from build123d import *

# Parameters (mm, degrees)
F0_W      = 16
F0_H      = 16
F1_DEPTH  = 16
F2_R      = 1
F4_R      = 1.5
F5_DEPTH  = 1
F3_R      = 1.5
F6_DEPTH  = 1
F7_R      = 1.5
F8_DEPTH  = 1
F9_R      = 1.5
F10_DEPTH = 1
F12_R     = 1.5
F13_DEPTH = 1
F11_R     = 1.5
F14_DEPTH = 1


with BuildPart() as f1:
    # F0 (on Top) → F1 (new body)
    with BuildSketch(Plane.XY):
        Rectangle(F0_W, F0_H)
    extrude(amount=F1_DEPTH)

    # F2
    f2_edges = [f1.edges().sort_by_distance(p)[0] for p in [
        (8, 0, 0),
        (8, 8, 8),
        (8, -8, 8),
        (8, 0, 16),
        (-8, 0, 16),
        (-8, 0, 0),
        (-8, -8, 8),
        (-8, 8, 8),
        (0, -8, 16),
        (0, -8, 0),
        (0, 8, 0),
        (0, 8, 16),
    ]]
    fillet(f2_edges, radius=F2_R)

    # F4 (on face) → F5 (cut)
    with BuildSketch(Plane.XY.offset(16)):
        with Locations((3.670213, -3.041311)):
            Circle(F4_R)
        with Locations((3.670213, 2.806282)):
            Circle(F4_R)
        with Locations((0, 2.806282)):
            Circle(F4_R)
        with Locations((-3.749967, 2.806282)):
            Circle(F4_R)
        with Locations((-3.749967, -3.041311)):
            Circle(F4_R)
        with Locations((0, -3.041311)):
            Circle(F4_R)
    extrude(amount=-F5_DEPTH, mode=Mode.SUBTRACT)

    # F3 (on face) → F6 (cut)
    with BuildSketch(Plane(origin=(0, 0, 0), x_dir=(1, 0, 0), z_dir=(0, 0, -1))):
        Circle(F3_R)
    extrude(amount=-F6_DEPTH, mode=Mode.SUBTRACT)

    # F7 (on face) → F8 (cut)
    with BuildSketch(Plane.XZ.offset(8)):
        with Locations((-3.057017, 4.979474)):
            Circle(F7_R)
        with Locations((2.599712, 4.979474)):
            Circle(F7_R)
        with Locations((-3.057017, 11.075789)):
            Circle(F7_R)
        with Locations((2.599712, 11.075789)):
            Circle(F7_R)
    extrude(amount=-F8_DEPTH, mode=Mode.SUBTRACT)

    # F9 (on face) → F10 (cut)
    with BuildSketch(Plane(origin=(-8, 0, 0), x_dir=(0, -1, 0), z_dir=(-1, 0, 0))):
        with Locations((-2.80434, 5.19566)):
            Circle(F9_R)
        with Locations((2.57599, 10.57599)):
            Circle(F9_R)
    extrude(amount=-F10_DEPTH, mode=Mode.SUBTRACT)

    # F12 (on face) → F13 (cut)
    with BuildSketch(Plane.YZ.offset(8)):
        with Locations((0, 8)):
            Circle(F12_R)
        with Locations((3.151538, 4.848462)):
            Circle(F12_R)
        with Locations((-3.246599, 11.246599)):
            Circle(F12_R)
        with Locations((-2.871442, 5.128558)):
            Circle(F12_R)
        with Locations((3.205944, 11.205944)):
            Circle(F12_R)
    extrude(amount=-F13_DEPTH, mode=Mode.SUBTRACT)

    # F11 (on face) → F14 (cut)
    with BuildSketch(Plane(origin=(0, 8, 0), x_dir=(-1, 0, 0), z_dir=(0, 1, 0))):
        with Locations((-3.412174, 11.412174)):
            Circle(F11_R)
        with Locations((3.286976, 4.713024)):
            Circle(F11_R)
        with Locations((0, 8)):
            Circle(F11_R)
    extrude(amount=-F14_DEPTH, mode=Mode.SUBTRACT)


solid = f1.part
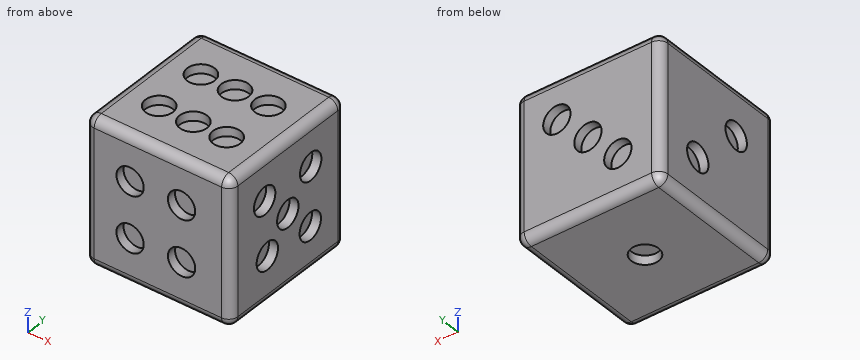
Could you check a few things on this model? Use its own coordinates, in mm. Coordinates: 2 decimals unless noted, no trailing zeros. Order: outer loops, then holes, each group sorted by start corner. A loop starts at its lowest first (then second) coordinate and runs counter-clockwise, first axis right, second up.
Q1. Will these pins go through, and if not, where does the flat tip stop? pin 1 (0.9 mm diameter, centred on y = 2.5, z = 4.5, fed in from -X); pin 2 (0.9 mm diameter, centred on x = -0.5, y = 2.5, fed in from +Z).
Q2. Suppose I cut it at C-C on y = 0. Please give me the cut outline in (x, z).
Q3. Suppose I cut it at B-B on x = 0. Please give me the cut outline in (y, z).
Q4. Suppose I cut it at A-A on z = 8. Please give me the cut outline in (x, y).
Q5. Please list where these lines run through material, in increasing order: L1, parallel to Z at x = -3.5, y = -4.25; L2, parallel to Y at x = 1.5, z = 11.25; L3, parallel to X at y = 0.5, z = 7.
Q6. Suppose I cut it at D-D on x = 7.25. Please give me the cut outline in (y, z).
Answer:
1. pin 1: stops at x = -7
1. pin 2: stops at z = 15
2. outline: (-8, 1) arc R1 ccw to (-7, 0) - (-1.5, 0) - (-1.5, 1) - (1.5, 1) - (1.5, 0) - (7, 0) arc R1 ccw to (8, 1) - (8, 6.5) - (7, 6.5) - (7, 9.5) - (8, 9.5) - (8, 15) arc R1 ccw to (7, 16) - (-7, 16) arc R1 ccw to (-8, 15) - close
3. outline: (-8, 1) arc R1 ccw to (-7, 0) - (-1.5, 0) - (-1.5, 1) - (1.5, 1) - (1.5, 0) - (7, 0) arc R1 ccw to (8, 1) - (8, 6.5) - (7, 6.5) - (7, 9.5) - (8, 9.5) - (8, 15) arc R1 ccw to (7, 16) - (4.31, 16) - (4.31, 15) - (1.31, 15) - (1.31, 16) - (-1.54, 16) - (-1.54, 15) - (-4.54, 15) - (-4.54, 16) - (-7, 16) arc R1 ccw to (-8, 15) - close
4. outline: (-8, -7) arc R1 ccw to (-7, -8) - (7, -8) arc R1 ccw to (8, -7) - (8, -1.5) - (7, -1.5) - (7, 1.5) - (8, 1.5) - (8, 7) arc R1 ccw to (7, 8) - (1.5, 8) - (1.5, 7) - (-1.5, 7) - (-1.5, 8) - (-7, 8) arc R1 ccw to (-8, 7) - close
5. L1: z = 0 to 15
5. L2: y = -7 to 8
5. L3: x = -8 to 7
6. outline: (-7.97, 1) arc R0.97 ccw to (-7, 0.03) - (7, 0.03) arc R0.97 ccw to (7.97, 1) - (7.97, 15) arc R0.97 ccw to (7, 15.97) - (-7, 15.97) arc R0.97 ccw to (-7.97, 15) - close; hole circle Ø3 at (-3.25, 11.25); hole circle Ø3 at (-2.87, 5.13); hole circle Ø3 at (0, 8); hole circle Ø3 at (3.15, 4.85); hole circle Ø3 at (3.21, 11.21)
